from build123d import *

# Parameters (mm, degrees)
F0_R     = 177.8
F1_DEPTH = 152.4
F2_R     = 44.45
F3_DEPTH = 209.55
F4_SIZE  = 38.1
F5_T     = -6.35
F6_R     = 132.6910727627
F7_DEPTH = 6.35


with BuildPart() as f1:
    # F0 (on Top) → F1 (new body)
    with BuildSketch(Plane.XY):
        Circle(F0_R)
    extrude(amount=F1_DEPTH)

    # F2 (on face) → F3 (join)
    with BuildSketch(Plane(origin=(0, 0, 0), x_dir=(1, 0, 0), z_dir=(0, 0, -1))):
        with Locations((76.2, 0)):
            Circle(F2_R)
        with Locations((0, 76.2)):
            Circle(F2_R)
        with Locations((-76.2, 0)):
            Circle(F2_R)
    extrude(amount=F3_DEPTH)

    # F4
    f4_edges = [f1.edges().sort_by_distance(p)[0] for p in [
        (-177.8, 0, 0),
    ]]
    chamfer(f4_edges, length=F4_SIZE)

    # F5
    f5_openings = [f1.faces().sort_by_distance(p)[0] for p in [
        (0, 0, 152.4),
    ]]
    offset(amount=F5_T, openings=f5_openings, kind=Kind.INTERSECTION)

    # F6 (on face) → F7 (cut)
    with BuildSketch(Plane(origin=(0, 0, -209.55), x_dir=(1, 0, 0), z_dir=(0, 0, -1))):
        Circle(F6_R)
    extrude(amount=-F7_DEPTH, mode=Mode.SUBTRACT)


solid = f1.part
Verification items for the finished model (mm, model axes). A direction names the side the tool comes from. Give positions to 0.01 mm unless a question says otherwise; leave off trailing zeros. Loops run counter-clockwise (first coordinate to the right, second up) from the corner with the lowest first, then second, coordinate; pieces in that order, holes last. Notation, with made-up numbers: (75.5, 39.5) - (107.5, 39.5) arc R24 cw to (107.5, 74.5) - close; hole circle Ø11 at (89, -21.75). An arc over 180 degrees is marked (long way). Write item = value, one per line. Start each with the question number.
Q1. Cross-section at B-B, the plane z = -16. Enter the section's corners in (x, y).
Q2. Cross-section at C-C, the plane y = 27.5. State how many separate pieces and enclosed holes the cut face has, and give its area (3 significant figures).
Q3. Cross-section at A-A, the plane x = 0. Enter the section's corners in (y, z), and give its area (3 significant figures).
Q4. Mould release check, pull along Y, two halves, no side actions. Record for faces 4 (the face through (-2, 2, 6.35)), 5 (the face through (-93, 146, 152.4)), 6 (the face through (-110.1, -84.42, 8.02)), 7 (the face through (-30.685, -138.184, 1.85)): released by +Y, released by -Y, zero draft, split by the parting line, or undercut.
Q5. Depth check by flat-ended pin: P1, Ø12, axis at y = 53.5, z = -108.5, coming from the -X side; P2, Ø12, axis at x = 91, z = 63, coming from the -Y side; P3, Ø2, axis at x = 71.5, z = 91.5, coming from the -Y side; P4, Ø1, axis at x = -22, y = -121.5, coming from the -Z side. Enter the tip coordinate at first touch or a pass-through.
Q6. Tool access check on faces 1 (the face through (169.59, 53.41, 94.45)), 2 (the face through (-120.607, -1.954, -100.178)), 3 (the face through (-22.32, 169.99, 95.78)). Record the directions out of +Z, -Z, +X, -X, +Y, -Y that give a thin tool (end or side, any length) a straight path to the whole face; none if there is none.
Q7. Thickness scan on line 1 (Y direction, x = -76.2, z = -74.5); line 2 (X direction, y = 12, z = -96); line 3 (Y direction, x = 0, z = -156). Record the ranges inside material, lowest first.
Answer key:
q1.outline = circle Ø88.9 at (-76.2, 0); circle Ø88.9 at (0, -76.2); circle Ø88.9 at (76.2, 0); hole circle Ø76.2 at (-76.2, 0); hole circle Ø76.2 at (0, -76.2); hole circle Ø76.2 at (76.2, 0)
q2.separate_pieces = 3
q2.enclosed_holes = 0
q2.area = 10,100 mm^2
q3.outline = (-177.8, 38.1) - (-139.7, 0) - (-120.65, 0) - (-120.65, -203.2) - (-114.3, -203.2) - (-114.3, 6.35) - (-137.07, 6.35) - (-171.45, 40.73) - (-171.45, 152.4) - (-177.8, 152.4) - close; (-38.1, -203.2) - (-31.75, -203.2) - (-31.75, 0) - (139.7, 0) - (177.8, 38.1) - (177.8, 152.4) - (171.45, 152.4) - (171.45, 40.73) - (137.07, 6.35) - (-38.1, 6.35) - close
q3.area = 5,940 mm^2
q4.face_4 = undercut
q4.face_5 = zero draft
q4.face_6 = undercut
q4.face_7 = split by the parting line
q5.P1 = through
q5.P2 = -156.17
q5.P3 = -163.23
q5.P4 = 0
q6.face_1 = +Z, -Z
q6.face_2 = -Z
q6.face_3 = +Z
q7.line_1 = -44.45 to -38.1, 38.1 to 44.45
q7.line_2 = -119 to -112.36, -40.04 to -33.4, 33.4 to 40.04, 112.36 to 119
q7.line_3 = -120.65 to -114.3, -38.1 to -31.75
